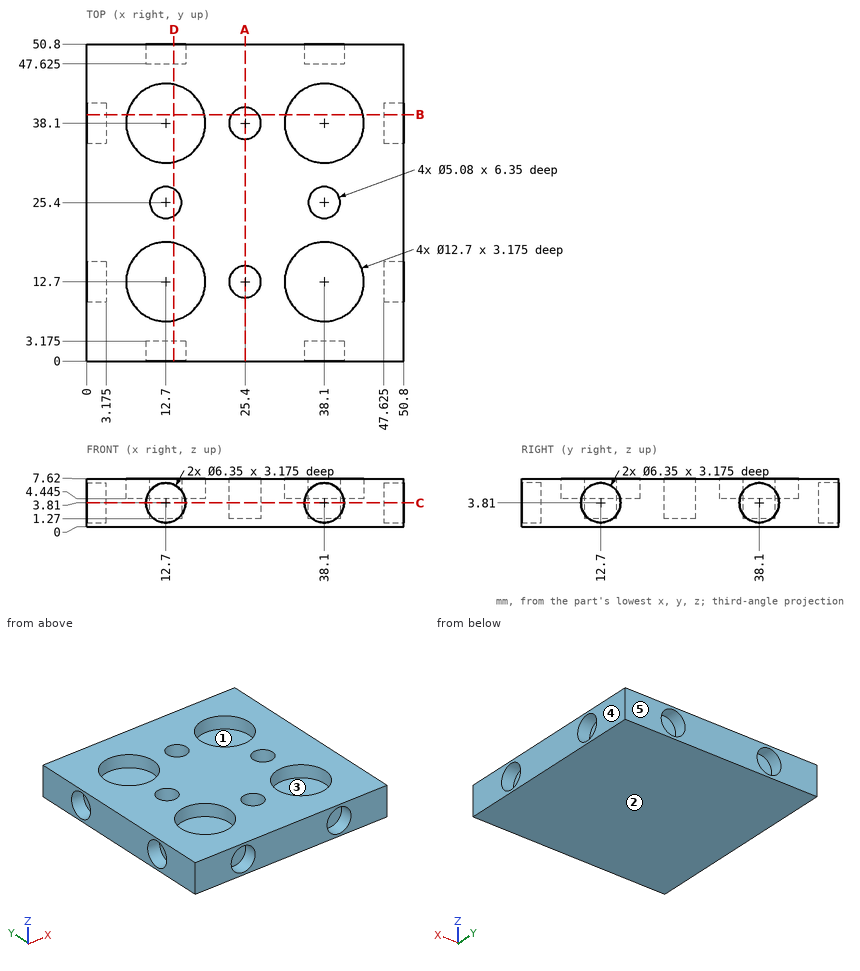
Could you check a few things on this drawing? It's one solid part, dimensions in mm from its lowest x, y, z. A direction names the side the tool comes from. Coordinates: 2 decimals unless noted, no trailing zeros. Order: outer loops, then holes, each group sorted by start corner. A loop starts at its lowest first (then second) coordinate and runs counter-clockwise, first axis right, second up.
1. I need wall thicknesses on line 1 (Y direction, x = 12.7, z = 7.05); line 2 (Y direction, x = 38.1, z = 5.7) (3 decimals); line 3 (Y direction, x = 12.7, z = 2.5) (3 decimals). Which ranges of each line are inside material? Lowest first, please.
2. For the marked faces 1 and 2, which set-ups out of +Z, -Z, +X, -X, +Y, -Y let a thin tool reach every point of the face, with its end or its side?
3. If we section it at A-A (x = 25.4): Please give me the cut outline in (y, z).
4. Thinking about a two-plate mould opening in Y: for the marked faces 3, 4 and 5, which applies, +Y half, -Y half, draft (parallel to the pull), parting line (faces both ways), or undercut?
5. If we section it at D-D (x = 14): Please give me the cut outline in (y, z) (1 decimal), then the cut area to 3 significant figures.
6. I'm going to push flat-ended pins straight in: pin 1 (10 mm diameter, centred on x = 12.7, y = 12.7, fed in from +Z) (3 decimals); pin 2 (1.5 mm diameter, centred on x = 26, y = 38, fed in from +Z); pin 3 (1.9 mm diameter, centred on x = 37, z = 2, fed in from -Y) (3 decimals). Where does each tip first touch, or does it pass through?
7. If we section it at C-C (z = 3.81): Give the number of separate pieces and of enclosed holes in the cut face, then the cut area to 3 significant figures.
8. If we section it at B-B (y = 39.5): Please give me the cut outline in (x, z) (3 decimals).
Entries:
1. line 1: y = 0 to 6.35, 19.05 to 22.86, 27.94 to 31.75, 44.45 to 50.8
1. line 2: y = 3.175 to 6.35, 19.05 to 22.86, 27.94 to 31.75, 44.45 to 47.625
1. line 3: y = 3.175 to 22.86, 27.94 to 47.625
2. face 1: +Z
2. face 2: -Z, +X, -X, +Y, -Y
3. outline: (0, 0) - (50.8, 0) - (50.8, 7.62) - (40.64, 7.62) - (40.64, 1.27) - (35.56, 1.27) - (35.56, 7.62) - (15.24, 7.62) - (15.24, 1.27) - (10.16, 1.27) - (10.16, 7.62) - (0, 7.62) - close
4. face 3: undercut
4. face 4: draft
4. face 5: +Y half
5. outline: (0, 0) - (50.8, 0) - (50.8, 0.9) - (47.6, 0.9) - (47.6, 6.7) - (50.8, 6.7) - (50.8, 7.6) - (44.3, 7.6) - (44.3, 4.4) - (31.9, 4.4) - (31.9, 7.6) - (27.6, 7.6) - (27.6, 1.3) - (23.2, 1.3) - (23.2, 7.6) - (18.9, 7.6) - (18.9, 4.4) - (6.5, 4.4) - (6.5, 7.6) - (0, 7.6) - (0, 6.7) - (3.2, 6.7) - (3.2, 0.9) - (0, 0.9) - close
5. area: 244 mm2
6. pin 1: stops at z = 4.445
6. pin 2: stops at z = 1.27
6. pin 3: stops at y = 3.175
7. separate pieces: 1
7. enclosed holes: 4
7. area: 2,340 mm2
8. outline: (0, 0) - (50.8, 0) - (50.8, 0.96) - (47.625, 0.96) - (47.625, 6.66) - (50.8, 6.66) - (50.8, 7.62) - (44.294, 7.62) - (44.294, 4.445) - (31.906, 4.445) - (31.906, 7.62) - (27.519, 7.62) - (27.519, 1.27) - (23.281, 1.27) - (23.281, 7.62) - (18.894, 7.62) - (18.894, 4.445) - (6.506, 4.445) - (6.506, 7.62) - (0, 7.62) - (0, 6.66) - (3.175, 6.66) - (3.175, 0.96) - (0, 0.96) - close
